Part model, mm, in its own coordinate system. A direction names the side the tool comes from. Coordinates: 2 decimals unless noted, no trailing zeros. Write each loop counter-clockwise with the first axis right and the second up, starting at its lowest first coordinate (ties: lowest second). Pieces come first, ordered by that corner, then holes. Notation, with made-up numbers: (23, -3) - (29, -3) arc R28 ccw to (29, 21) - close; hole circle Ø3 at (1, -8). An arc over 180 degrees is marked (long way). Write each question's results on one line, items separated by ' | '.
from build123d import *

# Parameters (mm, degrees)
F0_W     = 3
F0_H     = 8.4
F1_DEPTH = 3
F2_DEPTH = 15


with BuildPart() as f1:
    # F0 (on Top) → F1 (new body)
    with BuildSketch(Plane.XY):
        Polygon((-3, 0), (0, 0), (5, 0), (5, -2.1), (9, -2.1), (9, 1), (13, 1), (13, 4), (-3, 4), align=None)
        with Locations((-1.5, -4.2)):
            Rectangle(F0_W, F0_H)
        Polygon((5, -8.4), (0, -8.4), (-3, -8.4), (-3, -12.4), (13, -12.4), (13, -9.4), (9, -9.4), (9, -6.3), (5, -6.3), align=None)
        Polygon((5, 0), (0, 0), (0, -8.4), (5, -8.4), (5, -6.3), (9, -6.3), (9, -9.4), (13, -9.4), (13, 1), (9, 1), (9, -2.1), (5, -2.1), align=None)
    extrude(amount=-F1_DEPTH)

    # F0 (on Top) → F2 (join)
    with BuildSketch(Plane.XY):
        Polygon((-3, 0), (0, 0), (5, 0), (5, -2.1), (9, -2.1), (9, 1), (13, 1), (13, 4), (-3, 4), align=None)
        Polygon((5, -8.4), (0, -8.4), (-3, -8.4), (-3, -12.4), (13, -12.4), (13, -9.4), (9, -9.4), (9, -6.3), (5, -6.3), align=None)
        with Locations((-1.5, -4.2)):
            Rectangle(F0_W, F0_H)
    extrude(amount=F2_DEPTH)


solid = f1.part
(1) Saw through at C-C on y = -1.25. Write the cut outline in (x, z).
Return value:
outline: (-3, -3) - (13, -3) - (13, 0) - (9, 0) - (9, 15) - (5, 15) - (5, 0) - (0, 0) - (0, 15) - (-3, 15) - close
(2) Saw through at B-B on x = 3.25. Write the cut outline in (y, z).
Return value:
outline: (-12.4, -3) - (4, -3) - (4, 15) - (0, 15) - (0, 0) - (-8.4, 0) - (-8.4, 15) - (-12.4, 15) - close
(3) Flat gauge pins, fed straight in: P1, Ø2.5, axis at y = 0, z = 6, coming from the +X side; P2, Ø4, axis at y = -4, z = 9, coming from the +X side. Where does each tip first touch, or does it go through?
Return value:
P1: stops at x = 13 | P2: stops at x = 9
(4) Saw through at A-A on z = 12.5. Write the cut outline in (x, y), then the cut area to 3 significant figures.
Return value:
outline: (-3, -12.4) - (13, -12.4) - (13, -9.4) - (9, -9.4) - (9, -6.3) - (5, -6.3) - (5, -8.4) - (0, -8.4) - (0, 0) - (5, 0) - (5, -2.1) - (9, -2.1) - (9, 1) - (13, 1) - (13, 4) - (-3, 4) - close | area: 162 mm^2
(5) Wall check: line 1 (Y direction, x = 9.75, z = 2.25); line 2 (Y direction, x = 2.75, z = 1.5); line 3 (X direction, y = -7.75, z = 12.5). Give the ranges that are in metal, low to high. Write a range as from..to.
Return value:
line 1: y = -12.4..-9.4, 1..4 | line 2: y = -12.4..-8.4, 0..4 | line 3: x = -3..0, 5..9
(6) 3-axis set-ups, long thin cutter, end or side, ignore diameter. For faces 5 (the flat face through (7, -6.3, 7)), 6 (the flat face through (-0.4, -4.1, 15)), 7 (the flat face through (3, -8.4, 7)): which of +Z, -Z, +X, -X, +Y, -Y reach the whole face in a straight line?
Return value:
face 5: +Z, +X | face 6: +Z, +X, -X, +Y, -Y | face 7: +Z
(7) Two-plate mould, pull along X, no slides. Class faces 1 (the flat face through (-3, -4, 6)), 2 (the flat face through (13, 1.2, 6.1)), 3 (the flat face through (11, 1, 7)), 4 (the flat face through (6, -4, 0)): released by +X, released by -X, zero draft, split by the parting line, or undercut.
Return value:
face 1: released by -X | face 2: released by +X | face 3: zero draft | face 4: undercut
(8) Saw through at D-D on x = 7. Write the cut outline in (y, z).
Return value:
outline: (-12.4, -3) - (4, -3) - (4, 15) - (-2.1, 15) - (-2.1, 0) - (-6.3, 0) - (-6.3, 15) - (-12.4, 15) - close
